For this review, take the finished solid that the model builds, in its own axes (mm). Face numbers are marked on the shaded views. A direction names the side the tool comes from. Coordinates: 2 decimals unless noted, no trailing zeros. One line per item, written item: value.
from build123d import *

# Parameters (mm, degrees)
BOSS_EXTRUDE1_DEPTH = 76.2
SKETCH2_W           = 6.985
SKETCH2_H           = 9.525
CUT_EXTRUDE1_DEPTH  = 119.84173867
CUT_EXTRUDE2_DEPTH  = 119.84173867
CUT_EXTRUDE3_DEPTH  = 119.84173867
FILLET1_R           = 2.54
CUT_EXTRUDE4_DEPTH  = 5.08
CUT_EXTRUDE6_DEPTH  = 15.113
FILLET2_R           = 0.508


with BuildPart() as part:
    # Sketch1 → Boss-Extrude1 (new body)
    with BuildSketch(Plane.XY):
        Polygon((-15.5575, 76.2), (15.5575, 76.2), (15.5575, -76.2), (7.845485509, -76.2), (9.525, -85.725), (-9.525, -85.725), (-7.845485509, -76.2), (-15.5575, -76.2), align=None)
    extrude(amount=BOSS_EXTRUDE1_DEPTH)

    # Sketch2 → Cut-Extrude1 (cut, through all)
    with BuildSketch(Plane(origin=(15.5575, 0, 0), x_dir=(0, 0, -1), z_dir=(1, 0, 0))):
        with Locations((-3.4925, -80.9625)):
            Rectangle(SKETCH2_W, SKETCH2_H)
    extrude(amount=-CUT_EXTRUDE1_DEPTH, mode=Mode.SUBTRACT)

    # Sketch3 → Cut-Extrude2 (cut, through all)
    with BuildSketch(Plane(origin=(15.5575, 0, 0), x_dir=(0, 0, -1), z_dir=(1, 0, 0))):
        with BuildLine():
            Line((-76.2, -85.725), (-76.2, -76.2))
            Line((-76.2, -76.2), (-76.2, 76.2))
            Line((-76.2, 76.2), (-6.541803462, 76.2))
            ThreePointArc((-6.541803462, 76.2), (-58.046669251, 2.411215556), (-76.2, -85.725))
        make_face()
        with BuildLine():
            Line((0, -76.2), (0, 67.75939176))
            ThreePointArc((0, 67.75939176), (-18.20597202, -4.22030412), (0, -76.2))
        make_face()
    extrude(amount=-CUT_EXTRUDE2_DEPTH, mode=Mode.SUBTRACT)

    # Sketch6 → Cut-Extrude3 (cut, through all)
    with BuildSketch(Plane(origin=(15.5575, 0, 0), x_dir=(0, 0, -1), z_dir=(1, 0, 0))):
        with BuildLine():
            ThreePointArc((-28.934409948, -61.883434575), (-23.879909813, -60.517759582), (-22.716254779, -55.412963136))
            ThreePointArc((-22.716254779, -55.412963136), (-30.753414225, -11.294498854), (-26.546552055, 33.352305435))
            ThreePointArc((-26.546552055, 33.352305435), (-49.181053892, -9.446405872), (-61.429710833, -56.286781256))
            ThreePointArc((-61.429710833, -56.286781256), (-59.737369376, -60.827463042), (-55.008021131, -61.883434575))
            ThreePointArc((-55.008021131, -61.883434575), (-41.971215539, -60.062859411), (-28.934409948, -61.883434575))
        make_face()
    extrude(amount=-CUT_EXTRUDE3_DEPTH, mode=Mode.SUBTRACT)

    # Fillet1
    fillet1_edges = [part.edges().sort_by_distance(p)[0] for p in [
        (0, 33.352305435, 26.546552055),
    ]]
    fillet(fillet1_edges, radius=FILLET1_R)

    # Sketch7 → Cut-Extrude4 (cut, symmetric)
    with BuildSketch(Plane(origin=(0, 0, 0), x_dir=(0, 0, -1), z_dir=(1, 0, 0))):
        with BuildLine():
            Line((-30.699128799, 4.016230293), (-17.981752538, 4.016230293))
            ThreePointArc((-17.981752538, 4.016230293), (-17.415803594, -19.667907964), (-13.161921654, -42.973769707))
            Line((-13.161921654, -42.973769707), (-26.264177108, -42.973769707))
            ThreePointArc((-26.264177108, -42.973769707), (-30.179968378, -19.639057999), (-30.699128799, 4.016230293))
        make_face()
    extrude(amount=CUT_EXTRUDE4_DEPTH, both=True, mode=Mode.SUBTRACT)

    # Sketch10 → Cut-Extrude6 (cut, symmetric)
    with BuildSketch(Plane(origin=(15.5575, 76.2, 6.541803462), x_dir=(-1, 0, 0), z_dir=(0, -0.7903999954772005, -0.6125910929401777))):
        Polygon((0, 5.170641427), (6.985, 5.170641427), (0, -3.655858573), align=None)
        Polygon((31.115, 5.170641427), (31.115, -3.655858573), (24.13, 5.170641427), align=None)
    extrude(amount=CUT_EXTRUDE6_DEPTH, both=True, mode=Mode.SUBTRACT)

    # Fillet2
    fillet2_edges = [part.edges().sort_by_distance(p)[0] for p in [
        (0, 76.2, 6.541803462),
        (-14.111333502, 74.930435776, 7.871138317),
        (14.111333502, 74.930435776, 7.871138317),
        (-15.5575, 5.090891194, 56.873019023),
        (15.5575, 5.090891194, 56.873019023),
    ]]
    fillet(fillet2_edges, radius=FILLET2_R)


solid = part.part
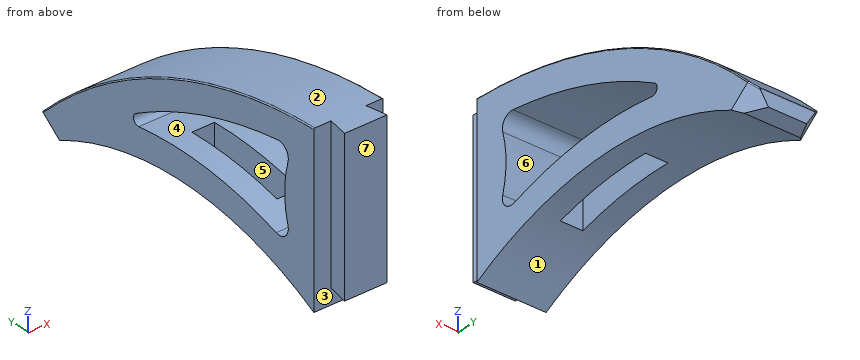
1. The part is to be moulded in two halves that separate along Z. For the marked faces 1, 2, 3 and 4, say which applies: pulls with the +Z half, pulls with the -Z half, needs draft (parallel to the pull), parting line crosses it, or undercut.
Return value:
face 1: pulls with the -Z half
face 2: pulls with the +Z half
face 3: needs draft
face 4: undercut
2. For the marked faces 5, 6 and 7, list the 3-axis set-ups (+Z, -Z, +X, -X, +Y, -Y) from which the entire face can be reached by the end or side of a thin tool; tool diameter is ignored.
Return value:
face 5: -Z
face 6: +X, -X
face 7: +Z, -Z, +X, -X, -Y
3. Take a section at A-A, the plane y = -8. Give the number of separate pieces and of enclosed holes in the cut face, and give its area (3 significant figures).
Return value:
separate pieces: 3
enclosed holes: 0
area: 689 mm2
4. To check wall thickness, follow probe 1 along Z at (x, y) = (2.5, -77.5) (3 decimals); probe 2 along Y at (x, z) = (-5, 5.5); probe 3 along Z at (x, y) = (4, 9). State the ranges of each line that lie inside material, in increasing order. Write a range as from..to.
Return value:
probe 1: z = 6.985..76.048
probe 2: y = -76.2..-64.93, 56.49..76.2
probe 3: z = 17.63..30.37, 40.96..55.08
5. Insertion check: pin 1 Ø4 at (x, y) = (-1, 54.5) entering from -Z; pin 2 Ø2 at (x, y) = (1, -28) entering from +Z; pin 3 Ø1 at (x, y) = (12, 51.5) entering from -Z. Each pin has a flat end and moves straight along its axis. Give the tip position at first contact, or say it passes through.
Return value:
pin 1: stops at z = 5.5
pin 2: stops at z = 68.87
pin 3: stops at z = 7.38
